Geometry check sheet. Reference: drawing and pictorial views, mm from the part's lowest x, y, z. Give positions to 0.01 mm unless a question says otherwise; leave off trailing zeros. Write each loop counter-clockwise with the first axis right and the second up, starting at its lowest first coordinate (ties: lowest second). Pieces come first, ordered by that corner, then holes. Notation, with made-up numbers: (34, 42) -> (93, 42) arc R5 cw to (93, 49) -> close; hole circle Ø2 at (-12.5, -35.75). An arc over 180 degrees is marked (long way). Return JSON: item names as keys, results as strings.
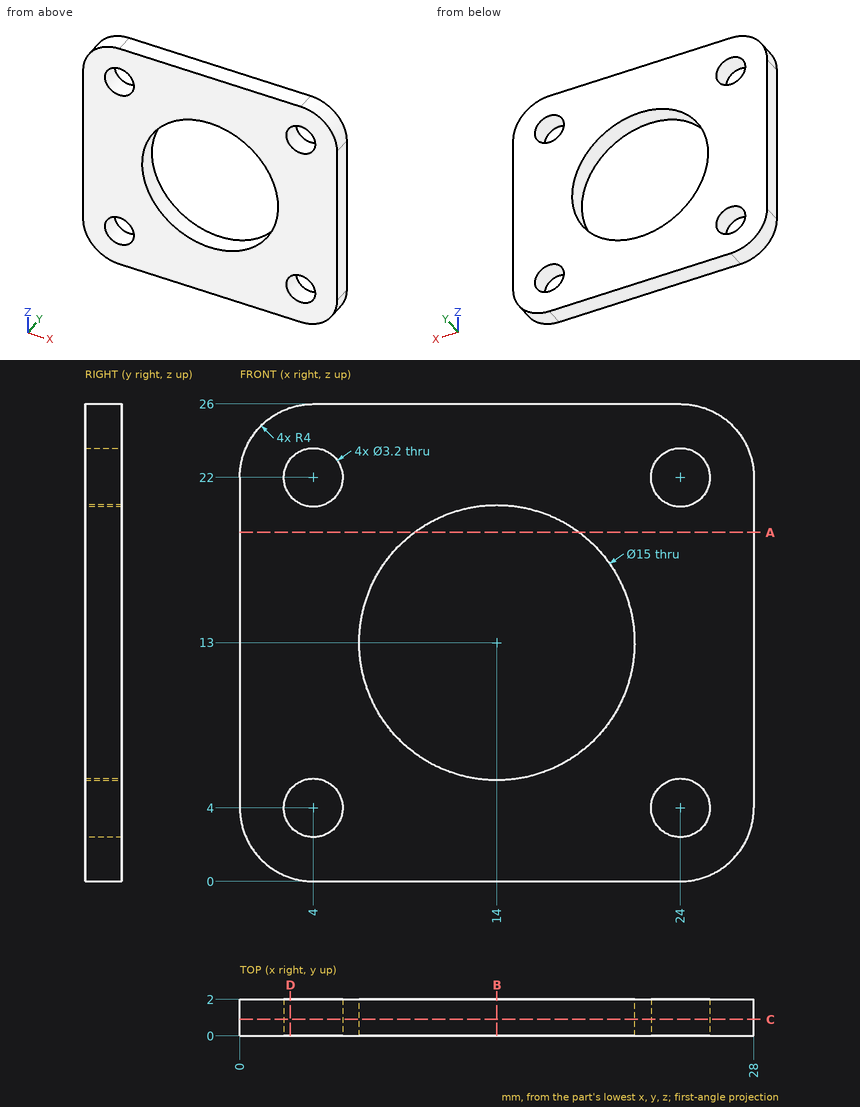
(1) Depth check by flat-ended pin: pin 1 Ø1 at (x, z) = (14, 19.5) entering from -Y. Enter the tip coordinate at first touch or a pass-through.
Reply:
{"pin 1": "through"}
(2) Cross-section at C-C on y = 0.9. Enter the section's corners in (x, z), then the cut area to 3 significant figures.
Reply:
{"outline": "(0, 4) arc R4 ccw to (4, 0) -> (24, 0) arc R4 ccw to (28, 4) -> (28, 22) arc R4 ccw to (24, 26) -> (4, 26) arc R4 ccw to (0, 22) -> close; hole circle Ø3.2 at (4, 4); hole circle Ø3.2 at (4, 22); hole circle Ø15 at (14, 13); hole circle Ø3.2 at (24, 4); hole circle Ø3.2 at (24, 22)", "area": "505 mm^2"}
(3) Thickness scan on L1, parallel to X at y = 0.5, z = 22; L2, parallel to X at y = 1.2, z = 3; L3, parallel to Z at x = 23, y = 0.5. Record the ranges inside material, lowest first.
Reply:
{"L1": "0 to 2.4, 5.6 to 22.4, 25.6 to 28", "L2": "0.13 to 2.75, 5.25 to 22.75, 25.25 to 27.87", "L3": "0 to 2.75, 5.25 to 20.75, 23.25 to 26"}
(4) Cross-section at A-A on z = 19. Enter the section's corners in (x, y).
Reply:
{"outline": "(0, 0) -> (9.5, 0) -> (9.5, 2) -> (0, 2) -> close; (18.5, 0) -> (28, 0) -> (28, 2) -> (18.5, 2) -> close"}
(5) Cross-section at B-B on x = 14. Enter the section's corners in (y, z).
Reply:
{"outline": "(0, 0) -> (2, 0) -> (2, 5.5) -> (0, 5.5) -> close; (0, 20.5) -> (2, 20.5) -> (2, 26) -> (0, 26) -> close"}
(6) Cross-section at D-D on x = 2.75. Enter the section's corners in (y, z).
Reply:
{"outline": "(0, 0.2) -> (2, 0.2) -> (2, 3) -> (0, 3) -> close; (0, 5) -> (2, 5) -> (2, 21) -> (0, 21) -> close; (0, 23) -> (2, 23) -> (2, 25.8) -> (0, 25.8) -> close"}
